```python
from build123d import *

# Parameters (mm, degrees)
SKETCH1_W           = 80
SKETCH1_H           = 39.6
BOSS_EXTRUDE1_DEPTH = 12
CUT_EXTRUDE2_REACH  = 92.068
SKETCH2_R           = 2.5
CUT_EXTRUDE3_DEPTH  = 20
FILLET1_R           = 1


with BuildPart() as part:
    # Sketch1 → Boss-Extrude1 (new body)
    with BuildSketch(Plane(origin=(0, 0, 0), x_dir=(1, 0, 0), z_dir=(0, 1, 0))):
        with Locations((40, 19.8)):
            Rectangle(SKETCH1_W, SKETCH1_H)
    extrude(amount=BOSS_EXTRUDE1_DEPTH)

    # Sketch2 → Cut-Extrude2 (cut, up to next)
    with BuildSketch(Plane(origin=(0, 0, -39.6), x_dir=(-1, 0, 0), z_dir=(0, 0, -1)), mode=Mode.PRIVATE) as cut_extrude2_sk1:
        with Locations((-38, 6)):
            Circle(SKETCH2_R)
    cut_extrude2_tool1 = extrude(cut_extrude2_sk1.sketch, amount=-CUT_EXTRUDE2_REACH, mode=Mode.PRIVATE) & part.part
    # Sketch2 → Cut-Extrude2 (cut, up to next)
    with BuildSketch(Plane(origin=(0, 0, -39.6), x_dir=(-1, 0, 0), z_dir=(0, 0, -1)), mode=Mode.PRIVATE) as cut_extrude2_sk2:
        with Locations((-73.8, 6)):
            Circle(SKETCH2_R)
    cut_extrude2_tool2 = extrude(cut_extrude2_sk2.sketch, amount=-CUT_EXTRUDE2_REACH, mode=Mode.PRIVATE) & part.part
    add(cut_extrude2_tool1.solids().sort_by_distance((38, 6, -39.6))[0], mode=Mode.SUBTRACT)
    add(cut_extrude2_tool2.solids().sort_by_distance((73.8, 6, -39.6))[0], mode=Mode.SUBTRACT)

    # Sketch3 → Cut-Extrude3 (cut)
    with BuildSketch(Plane(origin=(0, 0, -39.6), x_dir=(-1, 0, 0), z_dir=(0, 0, -1))):
        with BuildLine():
            Line((-63.4, 2), (-48.4, 2))
            ThreePointArc((-48.4, 2), (-45.571572875, 3.171572875), (-44.4, 6))
            Line((-44.4, 6), (-44.4, 12))
            Line((-44.4, 12), (-67.4, 12))
            Line((-67.4, 12), (-67.4, 6))
            ThreePointArc((-67.4, 6), (-66.228427125, 3.171572875), (-63.4, 2))
        make_face()
    extrude(amount=-CUT_EXTRUDE3_DEPTH, mode=Mode.SUBTRACT)

    # Fillet1
    fillet1_edges = [part.edges().sort_by_distance(p)[0] for p in [
        (80, 12, -19.8),
        (73.7, 12, -39.6),
        (22.2, 12, -39.6),
        (66.228427125, 3.171572875, -19.6),
        (67.4, 9, -19.6),
        (55.9, 12, -19.6),
        (67.4, 12, -29.6),
        (44.4, 9, -19.6),
        (44.4, 12, -29.6),
        (45.571572875, 3.171572875, -19.6),
        (55.9, 2, -19.6),
        (66.228427125, 3.171572875, -39.6),
        (55.9, 2, -39.6),
        (45.571572875, 3.171572875, -39.6),
        (44.4, 9, -39.6),
        (67.4, 9, -39.6),
        (0, 12, -19.8),
        (40, 12, 0),
        (0, 6, -39.6),
        (80, 6, -39.6),
        (80, 6, 0),
        (0, 6, 0),
    ]]
    fillet(fillet1_edges, radius=FILLET1_R)


solid = part.part
```
The listing builds one solid part. Answer for the finished solid, in the listing's coordinates (mm). A direction names the side the tool comes from. Coordinates: 2 decimals unless noted, no trailing zeros. Loops run counter-clockwise (first coordinate to the right, second up) from the corner with the lowest first, then second, coordinate; pieces in that order, holes last. Notation, with made-up numbers: M 47,57 L 100,57 A33 ccw 100,95 Z; hole C -31.5,71.25 d2. An arc over 180 degrees is marked long. Answer as CSV lines item,"result". Start each with the question number.
(1) The part is cut by section A-A (x = 73.8). Give the vertices of the cut face in (y, z), and give its area (3 significant figures).
(2) For faces 1 (the flat face through (56, 7, -19.6)), 2 (the flat face through (39, 3, 0)), determine the directions among +Z, -Z, +X, -X, +Y, -Y from which every point of the face is accessible in a straight line to the end or side of a thin tool.
(3) The part is cut by section C-C (y = 9.5). Give the vertices of the cut face in (x, z).
(4) The part is cut by section B-B (z = -8.5). Give the vertices of the cut face in (x, y).
(5) Find the intervals of material crossed by L1, parallel to X at y = 6.25, z = -16; L2, parallel to X at y = 8.25, z = -3.5; L3, parallel to X at y = 4, z = -25, in increasing order. Write a range as [from, to].
(6) The part is cut by section D-D (x = 61.5). Give the vertices of the cut face in (y, z).
(7) Given pin 1 (12 mm diameter, centred on x = 53.5, z = -29.5, fed in from +Y); pin 2 (4 mm diameter, centred on x = 73.8, y = 6, fed in from +Z); pin 3 (6 mm diameter, centred on x = 38, y = 6, fed in from +Z), each flat-ended and moving along its own axis, determine where each tip first touches the part or whether it passes through.
Determined:
1,outline,"M 0,-39.6 L 3.5,-39.6 L 3.5,0 L 0,0 Z; M 8.5,-39.6 L 11,-39.6 A1 ccw 12,-38.6 L 12,-1 A1 ccw 11,0 L 8.5,0 Z"
1,area,"277 mm2"
2,face 1,"-Z, +Y"
2,face 2,"+Z, +X, -X, +Y, -Y"
3,outline,"M 0,-38.6 A1 ccw 1,-39.6 L 43.4,-39.6 A1 ccw 44.4,-38.6 L 44.4,-20.6 A1 cw 45.4,-19.6 L 66.4,-19.6 A1 cw 67.4,-20.6 L 67.4,-38.6 A1 ccw 68.4,-39.6 L 79,-39.6 A1 ccw 80,-38.6 L 80,-1 A1 ccw 79,0 L 1,0 A1 ccw 0,-1 Z"
4,outline,"M 0,0 L 80,0 L 80,11 A1 ccw 79,12 L 1,12 A1 ccw 0,11 Z; hole C 38,6 d5; hole C 73.8,6 d5"
5,L1,"[0, 35.51], [40.49, 71.31], [76.29, 80]"
5,L2,"[0, 36.91], [39.09, 72.71], [74.89, 80]"
5,L3,"[0, 36.5], [39.5, 44.94], [66.86, 72.3], [75.3, 80]"
6,outline,"M 0,-39.6 L 1,-39.6 A1 ccw 2,-38.6 L 2,-20.6 A1 cw 3,-19.6 L 11,-19.6 A1 ccw 12,-18.6 L 12,-1 A1 ccw 11,0 L 0,0 Z"
7,pin 1,"y = 2.1"
7,pin 2,"through"
7,pin 3,"z = 0"
